Answer from the drawing. Dimensions are ordinates in mm from the lowest x, y and z of the part. Round coordinates to 2 decimals unless told otherwise and drop trailing zeros. Loops run counter-clockwise (first coordinate to the right, second up) from the corner with the lowest first, then second, coordinate; pieces in that order, holes last. Notation, with made-up numbers: (26.25, -20) - (76.25, -20) arc R26 cw to (76.25, -2) - close; hole circle Ø9 at (-22, 44.25). An arc over 180 degrees is marked (long way). Write item = value, one per line. Start each with the question number.
1) For a pull along X with two mould halves and no side action, classify the marked faces 1, 2, 3 and 4 as released by +X, released by -X, zero draft, split by the parting line, or undercut.
2) Straight lines are drawn through the part: line 1 along Y through (x, z) = (35.5, 37); line 2 along X through (y, z) = (35, 19.5); line 3 along Y through (x, z) = (39.5, 17). For each, find the intervals that lie inside material, in ascending order.
3) Section A-A, the plane y = 35 is taken. Determine the outline of the cut face in (x, z), and give its area (3 significant figures).
4) Section C-C, the plane z = 12 is taken. Determine the outline of the cut face in (x, y), and give its area (3 significant figures).
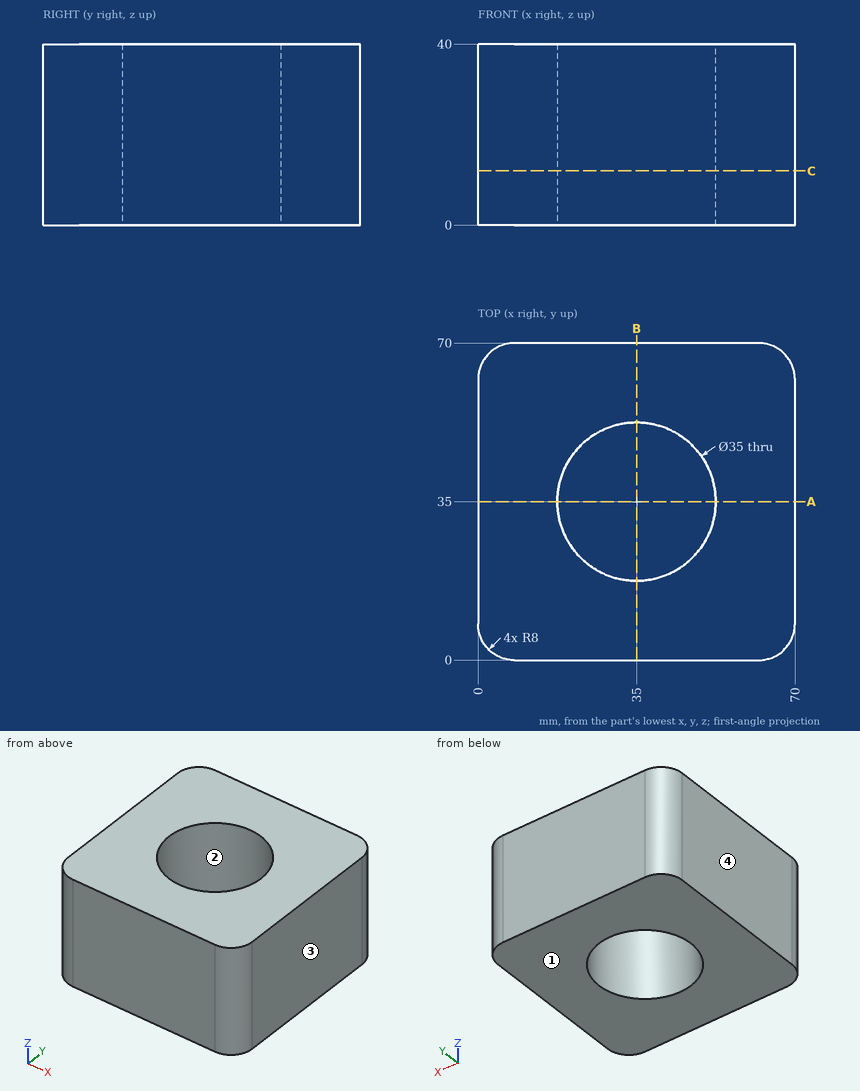
Geometry check:
q1.face_1 = zero draft
q1.face_2 = undercut
q1.face_3 = released by +X
q1.face_4 = released by -X
q2.line_1 = 0 to 17.51, 52.49 to 70
q2.line_2 = 0 to 17.5, 52.5 to 70
q2.line_3 = 0 to 18.09, 51.91 to 70
q3.outline = (0, 0) - (17.5, 0) - (17.5, 40) - (0, 40) - close; (52.5, 0) - (70, 0) - (70, 40) - (52.5, 40) - close
q3.area = 1,400 mm2
q4.outline = (0, 8) arc R8 ccw to (8, 0) - (62, 0) arc R8 ccw to (70, 8) - (70, 62) arc R8 ccw to (62, 70) - (8, 70) arc R8 ccw to (0, 62) - close; hole circle Ø35 at (35, 35)
q4.area = 3,880 mm2
